The listing builds one solid part. Answer for the finished solid, in the listing's coordinates (mm). Coordinates: 2 decimals unless noted, no trailing zeros. Order: outer loops, then holes, each group sorted by start corner. A loop starts at its lowest first (then second) coordinate and runs counter-clockwise, first axis right, second up.
```python
from build123d import *

# Parameters (mm, degrees)
SKETCH1_R           = 20.32
BOSS_EXTRUDE1_DEPTH = 25.4
SKETCH2_R           = 16.51
CUT_EXTRUDE1_DEPTH  = 39.353158931
SKETCH3_R           = 6.35
CUT_EXTRUDE2_DEPTH  = 39.353158931


with BuildPart() as part:
    # Sketch1 → Boss-Extrude1 (new body)
    with BuildSketch(Plane(origin=(0, 0, 0), x_dir=(1, 0, 0), z_dir=(0, 1, 0))):
        with Locations(Location((0, 0, 0), (0, 0, 270))):
            Circle(SKETCH1_R)
    extrude(amount=BOSS_EXTRUDE1_DEPTH)

    # Sketch2 → Cut-Extrude1 (cut, through all)
    with BuildSketch(Plane(origin=(0, 25.4, 0), x_dir=(1, 0, 0), z_dir=(0, 1, 0))):
        with Locations(Location((0, 0, 0), (0, 0, 270))):
            Circle(SKETCH2_R)
    extrude(amount=-CUT_EXTRUDE1_DEPTH, mode=Mode.SUBTRACT)

    # Sketch3 → Cut-Extrude2 (cut, through all)
    with BuildSketch(Plane.XY):
        Circle(SKETCH3_R)
    extrude(amount=-CUT_EXTRUDE2_DEPTH, mode=Mode.SUBTRACT)


solid = part.part
```
(1) Consider line 1 (Z direction, x = 0, y = 7.75); line 2 (Z direction, x = 4, y = 13). Determine where each line is inside the solid, lowest interval first.
(2) Find section C-C (y = 16.5). Write down the section's boundary in (x, z), and give its area (3 significant figures).
(3) Each of these flat-tipped pins is pushed along its axis until it touches: pin 1 Ø12 at (y, z) = (21, -7.5) entering from -X; pin 2 Ø1.5 at (y, z) = (3, -11.5) entering from +X; pin 3 Ø1.5 at (x, y) = (-3.5, 21.5) entering from -Z. Where does it stop, or does it pass through?
(4) The mould has two halves that part along X. Classify faces 1 (the face through (0.14, 6.35, -17.74)), 2 (the face through (2, 0, 17)), 3 (the face through (6.104, 12.522, 19.382)): released by +X, released by -X, zero draft, split by the parting line, or undercut.
(5) Find section D-D (y = 5.5). Write down the section's boundary in (x, z).
(6) Find section B-B (x = 0). Write down the section's boundary in (y, z), and give its area (3 significant figures).
(7) Find section A-A (z = 0). Write down the section's boundary in (x, y).
Findings below:
1. line 1: z = -20.32 to -16.51, 16.51 to 20.32
1. line 2: z = -19.92 to -16.02, 16.02 to 19.92
2. outline: circle Ø40.64 at (0, 0); hole circle Ø33.02 at (0, 0)
2. area: 441 mm2
3. pin 1: stops at x = -20.26
3. pin 2: stops at x = 17.24
3. pin 3: stops at z = -20.13
4. face 1: undercut
4. face 2: zero draft
4. face 3: split by the parting line
5. outline: (-3.17, -20.07) - (-3.17, -16.2) arc R16.51 cw (long way) to (3.17, -16.2) - (3.17, -20.07) arc R20.32 ccw (long way) to start
6. outline: (0, 16.51) - (25.4, 16.51) - (25.4, 20.32) - (0, 20.32) - close; (6.35, -20.32) - (25.4, -20.32) - (25.4, -16.51) - (6.35, -16.51) - close
6. area: 169 mm2
7. outline: (-20.32, 0) - (-16.51, 0) - (-16.51, 25.4) - (-20.32, 25.4) - close; (16.51, 0) - (20.32, 0) - (20.32, 25.4) - (16.51, 25.4) - close
